For this review, take the finished solid that the model builds, in its own axes (mm). Coordinates: 2 decimals unless noted, no trailing zeros. Order: outer loops, then holes, each group sorted by start corner. A loop starts at its lowest first (then second) coordinate and runs counter-clockwise, first axis right, second up. Notation, with made-up numbers: (33, 73.25) - (51, 73.25) arc R25 ccw to (51, 111.25) - close; hole circle Ø7 at (-38.75, 49.5). An arc over 180 degrees is marked (long way). One line per item, written item: value. Start each with the question number.
(1) Consider section A-A on x = 0. Write out the cut boundary in (y, z) (3 decimals), then the cut area to 3 significant figures.
(2) Clearance check with a flat-ended pin moving along its axis: pin 1 (2 mm diameter, centred on x = -36.67, z = -55.5, fed in from +Y). State where the tip first meets the part, or that it passes through.
(3) To check wall thickness, follow line 1 along X through (y, z) = (2.45, -35.5); line 2 along X through (y, z) = (2.55, -15.5). State the ranges of each line that lie inside material, in increasing order.
(4) Consider section B-B on y = 1.4. Count the separate pieces of the cut face and the enclosed holes in it, then the cut area to 3 significant figures.
(5) Mouldability with a two-part tool opening along Z and no side actions: class faces 1 (the flat face through (-1, 2, -71)), 2 (the flat face through (-1, 3.175, -1)), 3 (the cylindrical face through (53.705, 1.61, -47.429)) as released by +Z, released by -Z, zero draft, split by the parting line, or undercut.
```python
from build123d import *

# Parameters (mm, degrees)
SKETCH1_W           = 140
SKETCH1_H           = 142
BOSS_EXTRUDE1_DEPTH = 3.175
SKETCH2_R           = 6.25
SKETCH2_R_2         = 1.65
SKETCH2_R_3         = 1.25
CUT_EXTRUDE1_DEPTH  = 3.175
SKETCH4_R           = 2.1
CUT_EXTRUDE2_DEPTH  = 3.175


with BuildPart() as part:
    # Sketch1 → Boss-Extrude1 (new body)
    with BuildSketch(Plane(origin=(0, 0, 0), x_dir=(1, 0, 0), z_dir=(0, 1, 0))):
        Rectangle(SKETCH1_W, SKETCH1_H)
    extrude(amount=BOSS_EXTRUDE1_DEPTH)

    # Sketch2 → Cut-Extrude1 (cut)
    with BuildSketch(Plane(origin=(0, 3.175, 0), x_dir=(1, 0, 0), z_dir=(0, 1, 0))):
        with Locations(Location((-57.9286, 52.0357, 0), (0, 0, 270))):
            Circle(SKETCH2_R)
        with Locations(Location((-62.9286, 66.5357, 0), (0, 0, 270))):
            Circle(SKETCH2_R_2)
        with Locations(Location((-52.9286, 66.5357, 0), (0, 0, 90))):
            Circle(SKETCH2_R_2)
        with Locations(Location((-52.9286, 17.5357, 0), (0, 0, 270))):
            Circle(SKETCH2_R_2)
        with Locations(Location((-62.9286, 17.5357, 0), (0, 0, 90))):
            Circle(SKETCH2_R_2)
        with Locations(Location((52.9286, 17.5357, 0), (0, 0, 90))):
            Circle(SKETCH2_R_2)
        with Locations(Location((62.9286, 17.5357, 0), (0, 0, 270))):
            Circle(SKETCH2_R_2)
        with Locations(Location((57.9286, 52.0357, 0), (0, 0, 90))):
            Circle(SKETCH2_R)
        with Locations(Location((52.9286, 66.5357, 0), (0, 0, 270))):
            Circle(SKETCH2_R_2)
        with Locations(Location((62.9286, 66.5357, 0), (0, 0, 90))):
            Circle(SKETCH2_R_2)
        with Locations(Location((-36.666666667, 55.5, 0), (0, 0, 270))):
            Circle(SKETCH2_R_3)
        with Locations(Location((-36.666666667, 35.5, 0), (0, 0, 90))):
            Circle(SKETCH2_R_3)
        with Locations(Location((-63.333333333, 35.5, 0), (0, 0, 270))):
            Circle(SKETCH2_R_3)
        with Locations(Location((36.666666667, 35.5, 0), (0, 0, 270))):
            Circle(SKETCH2_R_3)
        with Locations(Location((63.333333333, 35.5, 0), (0, 0, 90))):
            Circle(SKETCH2_R_3)
        with Locations(Location((36.666666667, 55.5, 0), (0, 0, 90))):
            Circle(SKETCH2_R_3)
        with Locations(Location((63.333333333, -35.5, 0), (0, 0, 270))):
            Circle(SKETCH2_R_3)
        with Locations(Location((36.666666667, -35.5, 0), (0, 0, 90))):
            Circle(SKETCH2_R_3)
        with Locations(Location((63.333333333, -55.5, 0), (0, 0, 90))):
            Circle(SKETCH2_R_3)
        with Locations(Location((36.666666667, -55.5, 0), (0, 0, 270))):
            Circle(SKETCH2_R_3)
        with Locations(Location((-36.666666667, -35.5, 0), (0, 0, 270))):
            Circle(SKETCH2_R_3)
        with Locations(Location((-63.333333333, -35.5, 0), (0, 0, 90))):
            Circle(SKETCH2_R_3)
        with Locations(Location((-36.666666667, -55.5, 0), (0, 0, 90))):
            Circle(SKETCH2_R_3)
        with Locations(Location((-63.333333333, -55.5, 0), (0, 0, 270))):
            Circle(SKETCH2_R_3)
    extrude(amount=-CUT_EXTRUDE1_DEPTH, mode=Mode.SUBTRACT)

    # Sketch4 → Cut-Extrude2 (cut)
    with BuildSketch(Plane(origin=(0, 3.175, 0), x_dir=(1, 0, 0), z_dir=(0, 1, 0))):
        with Locations(Location((0, 30.525, 0), (0, 0, 270))):
            Circle(SKETCH4_R)
        with Locations(Location((26.435425451, 15.2625, 0), (0, 0, 270))):
            Circle(SKETCH4_R)
        with Locations(Location((26.435425451, -15.2625, 0), (0, 0, 270))):
            Circle(SKETCH4_R)
        with Locations(Location((0, -30.525, 0), (0, 0, 270))):
            Circle(SKETCH4_R)
        with Locations(Location((-26.435425451, -15.2625, 0), (0, 0, 270))):
            Circle(SKETCH4_R)
        with Locations(Location((-26.435425451, 15.2625, 0), (0, 0, 270))):
            Circle(SKETCH4_R)
    extrude(amount=-CUT_EXTRUDE2_DEPTH, mode=Mode.SUBTRACT)


solid = part.part
```
Geometry check:
1. outline: (0, -71) - (3.175, -71) - (3.175, -32.625) - (0, -32.625) - close; (0, -28.425) - (3.175, -28.425) - (3.175, 28.425) - (0, 28.425) - close; (0, 32.625) - (3.175, 32.625) - (3.175, 71) - (0, 71) - close
1. area: 424 mm^2
2. pin 1: passes through
3. line 1: x = -70 to -64.58, -62.08 to -37.92, -35.42 to 35.42, 37.92 to 62.08, 64.58 to 70
3. line 2: x = -70 to -28.52, -24.35 to 24.35, 28.52 to 70
4. separate pieces: 1
4. enclosed holes: 30
4. area: 19,400 mm^2
5. face 1: released by -Z
5. face 2: zero draft
5. face 3: undercut
